Can you work these out from the drawing? Everything is in mm from the part's minimum corner. A direction names the side the tool comes from. Coordinates: 2 decimals unless noted, no trailing zeros. Loops run counter-clockwise (first coordinate to the right, second up) from the corner with the lowest first, then second, coordinate; pieces in that order, holes last. Notation, with made-up numbers: (-24.5, 62.25) -> (17.5, 62.25) arc R30 cw to (17.5, 96.25) -> close; hole circle Ø8 at (-19.5, 9.25). An arc over 180 degrees is marked (long way). One line per question, with ' | ' between items.
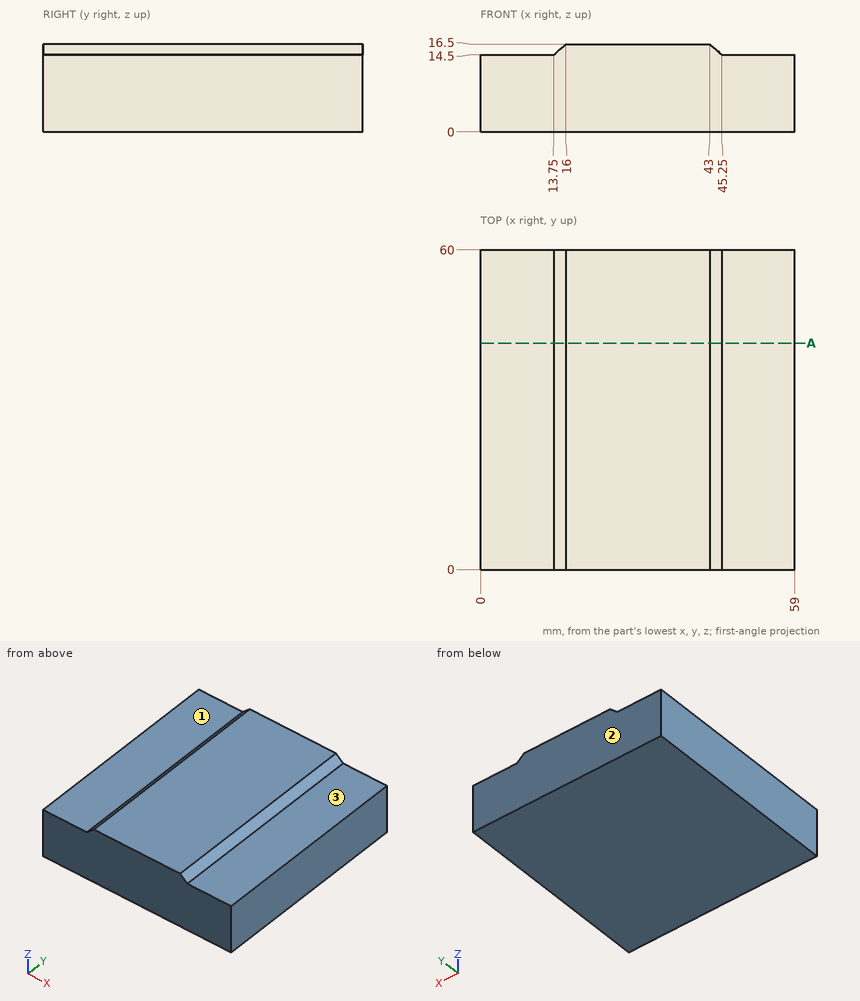
Q1. Imagine slicing it at A-A on y = 42.5. Write out the boundary of the cut face in (x, z), plus the area to 3 significant figures.
Values follow:
outline: (0, 0) -> (59, 0) -> (59, 14.5) -> (45.25, 14.5) -> (43, 16.5) -> (16, 16.5) -> (13.75, 14.5) -> (0, 14.5) -> close | area: 914 mm2
Q2. For pin 1 (4 mm diameter, centred on x = 52.5, y = 32, fed in from +Z), with a flat end and sliding along its axis, tell me the tip position at first contact or that it passes through.
Values follow:
pin 1: stops at z = 14.5
Q3. For the marked faces 1, 2 and 3, which set-ups out of +Z, -Z, +X, -X, +Y, -Y let a thin tool reach every point of the face, with its end or its side?
Values follow:
face 1: +Z, -X, +Y, -Y | face 2: +Z, -Z, +X, -X, +Y | face 3: +Z, +X, +Y, -Y
Q4. Please list where these lines run through material, in increasing order: L1, parallel to Z at x = 50, y = 38; L2, parallel to X at y = 7.5, z = 15. Write a range as [from, to].
Values follow:
L1: z = [0, 14.5] | L2: x = [14.31, 44.69]
